Can you work these out from the model? Positions are in its coordinate system, mm. Face numbers are marked on the shaded views. A direction names the side the tool comes from. Coordinates: 2 decimals unless noted, no trailing zeros. Order: outer loops, then holes, each group sorted by start corner. A loop starts at its lowest first (then second) coordinate and runs counter-clockwise, first axis right, second up. Notation, with made-up numbers: (54, -30) -> (112, -30) arc R20 cw to (112, -3) -> close; hole circle Ø7 at (18, -31.5). An arc over 180 degrees is marked (long way). Return JSON: item names as keys, results as strings. Group by question number.
1) For the marked faces 4, 5 and 6, which set-ups out of +Z, -Z, +X, -X, +Y, -Y let a thin tool reach every point of the face, with its end or its side?
2) For pin 1 (8 mm diameter, centred on x = 4.5, z = 8.5, fed in from +Y); pin 2 (2 mm diameter, centred on x = -29, y = 42, fed in from +Z); pin 3 (6 mm diameter, centred on x = 58.5, y = 59, fed in from +Z); pin 4 (3.5 mm diameter, centred on y = 54, z = 7.5, fed in from -X), each with a flat end and sliding along its axis, tell me the tip position at first contact or that it passes through.
3) If I drill on probe 1 along Y at (x, z) = (-69.25, 0.4); probe 2 along X at (y, z) = (91, 1.05); probe 3 along Y at (x, z) = (64, 12), over which ranges is the centre line in solid material (lowest first)? Write a range as from..to.
4) Thinking about a two-plate mould opening in Z: for the marked faces 1, 2 and 3, which applies, +Z half, -Z half, draft (parallel to the pull), parting line (faces both ways), or undercut?
5) If we section it at A-A, the plane y = 4: Please give me the cut outline in (x, z).
6) If we section it at B-B, the plane x = 69.25: Please give me the cut outline in (y, z).
7) If we section it at C-C, the plane z = 8.75: Please give me the cut outline in (x, y).
8) If we section it at D-D, the plane y = 38.5: Please give me the cut outline in (x, z), then the cut area to 3 significant figures.
from build123d import *

# Parameters (mm, degrees)
SKETCH001_W   = 15
SKETCH001_H   = 2
SKETCH001_W_2 = 16
SKETCH001_H_2 = 14
SKETCH001_W_3 = 12
SKETCH001_H_3 = 11
PAD001_DEPTH  = 20
SKETCH_W      = 146.5
SKETCH_H      = 95
SKETCH_R      = 1.8
PAD_DEPTH     = 2


with BuildPart() as pad001:
    # Sketch001 → Pad001 (new body)
    with BuildSketch(Plane(origin=(73.25, 0, 0), x_dir=(0, -1, 0), z_dir=(-1, 0, 0))):
        with Locations((-16.5, 3)):
            Rectangle(SKETCH001_W, SKETCH001_H)
        with Locations((-36, 9)):
            Rectangle(SKETCH001_W_2, SKETCH001_H_2)
        with Locations((-56, 7.5)):
            Rectangle(SKETCH001_W_3, SKETCH001_H_3)
    extrude(amount=PAD001_DEPTH)


with BuildPart() as fusion:
    # Sketch → Pad (new body)
    with BuildSketch(Plane.XY):
        with Locations((0, 47.5)):
            Rectangle(SKETCH_W, SKETCH_H)
        with Locations((-69.25, 91)):
            Circle(SKETCH_R, mode=Mode.SUBTRACT)
        with Locations((69.25, 91)):
            Circle(SKETCH_R, mode=Mode.SUBTRACT)
        with Locations((69.25, 4)):
            Circle(SKETCH_R, mode=Mode.SUBTRACT)
        with Locations((-69.25, 4)):
            Circle(SKETCH_R, mode=Mode.SUBTRACT)
    extrude(amount=PAD_DEPTH)

    # Fusion: union Pad001
    add(pad001.part)


solid = fusion.part
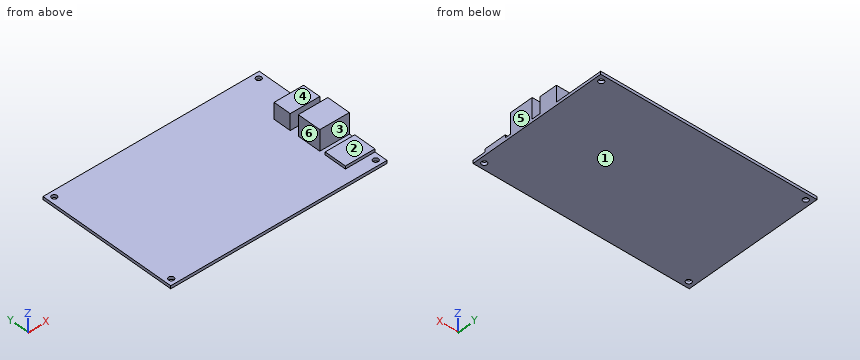
Result sheet:
{
 "1": {"face 4": "+Z, +X, -X, +Y", "face 5": "+Z, -Z, +X, +Y, -Y", "face 6": "+Z, -X, +Y, -Y"},
 "2": {"pin 1": "passes through", "pin 2": "stops at z = 2", "pin 3": "stops at z = 13", "pin 4": "stops at x = 53.25"},
 "3": {"probe 1": "y = 0..2.2, 5.8..89.2, 92.8..95", "probe 2": "x = -73.25..-71.05, -67.45..67.45, 71.05..73.25", "probe 3": "y = 28..44, 50..62"},
 "4": {"face 1": "-Z half", "face 2": "+Z half", "face 3": "draft"},
 "5": {"outline": "(-73.25, 0) -> (-71.05, 0) -> (-71.05, 2) -> (-73.25, 2) -> close; (-67.45, 0) -> (67.45, 0) -> (67.45, 2) -> (-67.45, 2) -> close; (71.05, 0) -> (73.25, 0) -> (73.25, 2) -> (71.05, 2) -> close"},
 "6": {"outline": "(0, 0) -> (2.2, 0) -> (2.2, 2) -> (0, 2) -> close; (5.8, 0) -> (89.2, 0) -> (89.2, 2) -> (62, 2) -> (62, 13) -> (50, 13) -> (50, 2) -> (44, 2) -> (44, 16) -> (28, 16) -> (28, 2) -> (24, 2) -> (24, 4) -> (9, 4) -> (9, 2) -> (5.8, 2) -> close; (92.8, 0) -> (95, 0) -> (95, 2) -> (92.8, 2) -> close"},
 "7": {"outline": "(53.25, 28) -> (73.25, 28) -> (73.25, 44) -> (53.25, 44) -> close; (53.25, 50) -> (73.25, 50) -> (73.25, 62) -> (53.25, 62) -> close"},
 "8": {"outline": "(-73.25, 0) -> (73.25, 0) -> (73.25, 16) -> (53.25, 16) -> (53.25, 2) -> (-73.25, 2) -> close", "area": "573 mm2"}
}
